Geometry check sheet. Reference: drawing and pictorial views, mm from the part's lowest x, y, z. A direction names the side the tool comes from. Give positions to 0.01 mm unless a question says otherwise; leave off trailing zeros. Order: outer loops, then holes, each group sorted by start corner. A loop starts at its lowest first (then second) coordinate and runs counter-clockwise, first axis right, second up.
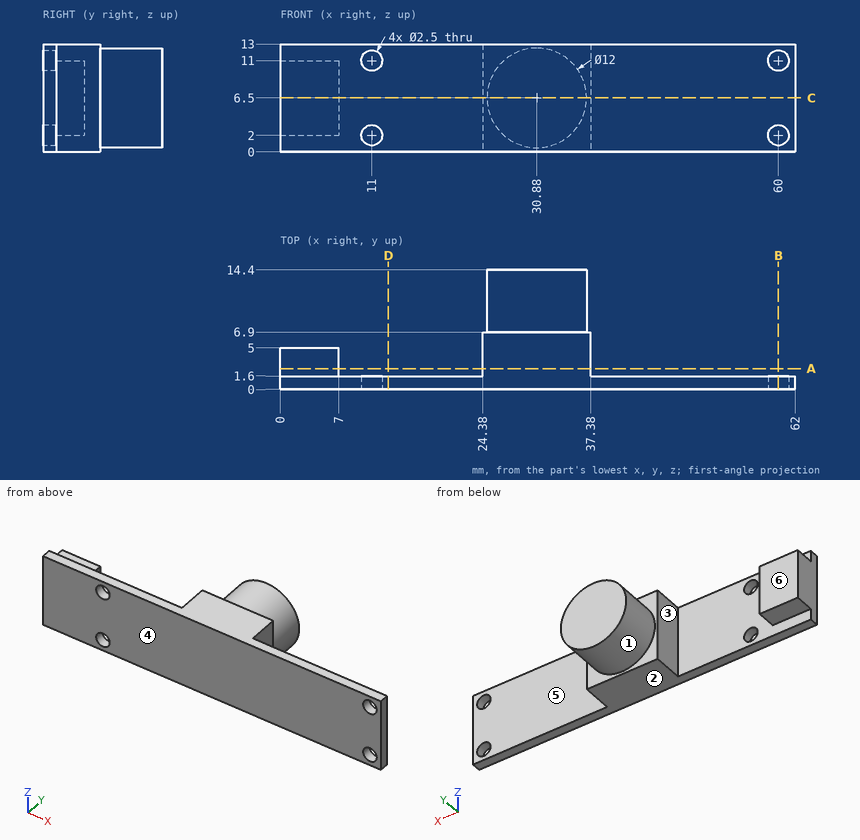
(1) Cross-section at D-D on x = 13. Enter the section's corners in (y, z).
Response values:
outline: (0, 0) - (1.6, 0) - (1.6, 13) - (0, 13) - close
(2) Cross-section at A-A on y = 2.5. Enter the section's corners in (x, z).
Response values:
outline: (0, 2) - (7, 2) - (7, 11) - (0, 11) - close; (24.38, 0) - (37.38, 0) - (37.38, 13) - (24.38, 13) - close
(3) Material ranges on L1, parallel to X at y = 0.45, z = 2; L2, parallel to Z at x = 60, y = 0.4; L3, parallel to X at y = 2, z = 3.75, recorded low to high.
Response values:
L1: x = 0 to 9.75, 12.25 to 58.75, 61.25 to 62
L2: z = 0 to 0.75, 3.25 to 9.75, 12.25 to 13
L3: x = 0 to 7, 24.38 to 37.38
(4) Release check for a two-part mould opening along X. For the marked faces 1, 2 and 3 record: released by +X, released by -X, zero draft, split by the parting line, or undercut.
Response values:
face 1: split by the parting line
face 2: zero draft
face 3: undercut
(5) Cross-section at C-C on z = 6.5. Enter the section's corners in (x, y).
Response values:
outline: (0, 0) - (62, 0) - (62, 1.6) - (37.38, 1.6) - (37.38, 6.9) - (36.88, 6.9) - (36.88, 14.4) - (24.88, 14.4) - (24.88, 6.9) - (24.38, 6.9) - (24.38, 1.6) - (7, 1.6) - (7, 5) - (0, 5) - close
(6) Set-up check for the marked faces 4, 5 and 6: record each of +Z, -Z, +X, -X, +Y, -Y from which the full face is reachable in a straight line by a thin tool's end or side.
Response values:
face 4: +Z, -Z, +X, -X, -Y
face 5: +Z, -Z, +X, +Y
face 6: +Z, -Z, -X, +Y
(7) Cross-section at B-B on x = 60. Enter the section's corners in (y, z), then the cut area to 3 significant figures.
Response values:
outline: (0, 0) - (1.6, 0) - (1.6, 0.75) - (0, 0.75) - close; (0, 3.25) - (1.6, 3.25) - (1.6, 9.75) - (0, 9.75) - close; (0, 12.25) - (1.6, 12.25) - (1.6, 13) - (0, 13) - close
area: 12.8 mm2
(8) Gauge pin test, flat ends, axial feed: pin 1 Ø1.5 at (x, z) = (11, 11) entering from +Y; pin 2 Ø6 at (y, z) = (3.5, 8.5) entering from -X; pin 3 Ø4 at (x, z) = (60, 2) entering from +Y; pin 4 Ø3.5 at (x, y) = (4.5, 3.5) entering from +Z. Record the tip position at first contact, or that the pin passes through.
Response values:
pin 1: passes through
pin 2: stops at x = 0
pin 3: stops at y = 1.6
pin 4: stops at z = 11
